Verification items for the finished model (mm, model axes). Face numbers are marked on the shaded views. Round coordinates to 2 decimals unless told otherwise and drop trailing zeros. Order: outer loops, then holes, each group sorted by start corner. A loop starts at its lowest first (then second) coordinate and runs counter-clockwise, first axis right, second up. Notation, with made-up numbers: M -11.75,-16.75 L 29.25,-16.75 A27 cw 29.25,22.25 Z; hole C 2,-24 d9. An arc over 180 degrees is marked long. Write item = value, one per line. Start each with the question number.
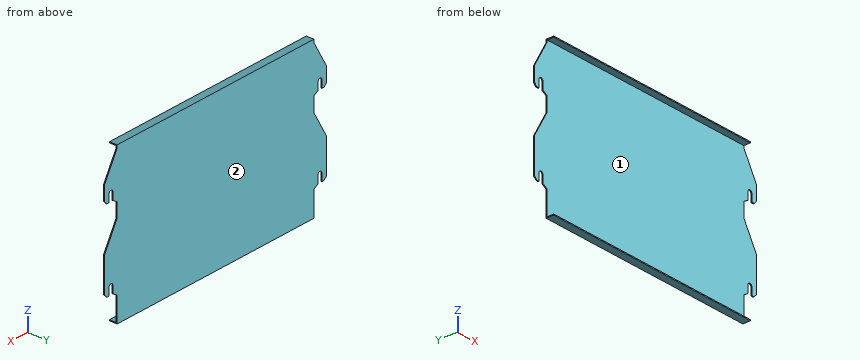
from build123d import *

# Parameters (mm, degrees)
EXTRUDE_THIN1_DEPTH = 132
CUT_EXTRUDE1_DEPTH  = 10


with BuildPart() as part:
    # Sketch1 → Extrude-Thin1 (new, symmetric)
    with BuildSketch(Plane(origin=(0, 0, 0), x_dir=(0, 0, -1), z_dir=(1, 0, 0))):
        Polygon((-80.5, -8), (-80.5, 0), (80.5, 0), (80.5, -8), (79.5, -8), (79.5, -1), (-79.5, -1), (-79.5, -8), align=None)
    extrude(amount=EXTRUDE_THIN1_DEPTH, both=True)

    # Sketch2 → Cut-Extrude1 (cut)
    with BuildSketch(Plane(origin=(0, 0, 0), x_dir=(1, 0, 0), z_dir=(0, 1, 0))):
        with BuildLine():
            Line((-117, 80.5), (-117, 54.5))
            Line((-117, 54.5), (-122, 51.5))
            Line((-122, 51.5), (-122, 43.5))
            ThreePointArc((-122, 43.5), (-124.25, 41.25), (-126.5, 43.5))
            Line((-126.5, 43.5), (-126.5, 51.5))
            Line((-126.5, 51.5), (-129, 51.5))
            Line((-129, 51.5), (-132, 48.5))
            Line((-132, 48.5), (-132, 12.5))
            Line((-132, 12.5), (-117, -14.5))
            Line((-117, -14.5), (-117, -29.5))
            Line((-117, -29.5), (-122, -32.5))
            Line((-122, -32.5), (-122, -40.5))
            ThreePointArc((-122, -40.5), (-124.25, -42.75), (-126.5, -40.5))
            Line((-126.5, -40.5), (-126.5, -32.5))
            Line((-126.5, -32.5), (-129.5, -32.5))
            Line((-129.5, -32.5), (-132, -35.5))
            Line((-132, -35.5), (-132, -50.5))
            Line((-132, -50.5), (-117, -77.5))
            Line((-117, -77.5), (-117, -80.5))
            Line((-117, -80.5), (-140, -80.5))
            Line((-140, -80.5), (-140, 80.5))
            Line((-140, 80.5), (-117, 80.5))
        make_face()
    cut_extrude1 = extrude(amount=-CUT_EXTRUDE1_DEPTH, mode=Mode.SUBTRACT)

    # Mirror1: Cut-Extrude1 across plane
    add(cut_extrude1.mirror(Plane(origin=(0, 0, 0), x_dir=(0, 0, 1), z_dir=(1, 0, 0))), mode=Mode.SUBTRACT)


solid = part.part
1) Scan lines: probe 1 along Z at (x, y) = (-25, -2.25); probe 2 along Y at (x, z) = (110.5, -18.5). Record each from-to range of solid material in increasing order.
2) Cross-section at B-B, the plane x = -28.5. Enter the section's corners in (y, z), then the cut area to 3 significant figures.
3) Cross-section at D-D, the plane z = -38. Enter the section's corners in (x, y), then the cut area to 3 significant figures.
4) Gauge pin test, flat ends, axial feed: P1, Ø5, axis at x = -89, z = -31.5, coming from the +Y side; P2, Ø3.5, axis at y = -5, z = 79.5, coming from the -X side; P3, Ø1.1, axis at y = -0.5, z = 23, coming from the +X side; P4, Ø0.5, axis at x = -128.5, y = -0.5, coming from the -Z side. Record the tip position at first contact, or that the pin passes through.
5) Cross-section at A-A, the plane y = -5.25. Enter the section's corners in (x, z), then the cut area to 3 significant figures.
6) Cross-section at C-C, the plane z = -67. Enter the section's corners in (x, y).
7) Release check for a two-part mould opening along Z. For the marked faces 1 and 2 record: pulls with the +Z half, pulls with the -Z half, needs draft (parallel to the pull), parting line crosses it, or undercut.
Geometry results:
q1.probe_1 = -80.5 to -79.5, 79.5 to 80.5
q1.probe_2 = -1 to 0
q2.outline = M -8,-80.5 L 0,-80.5 L 0,80.5 L -8,80.5 L -8,79.5 L -1,79.5 L -1,-79.5 L -8,-79.5 Z
q2.area = 175 mm^2
q3.outline = M -132,-1 L 132,-1 L 132,0 L -132,0 Z
q3.area = 264 mm^2
q4.P1 = 0
q4.P2 = -117
q4.P3 = 117
q4.P4 = -51.5
q5.outline = M -117,-80.5 L 117,-80.5 L 117,-79.5 L -117,-79.5 Z; M -117,79.5 L 117,79.5 L 117,80.5 L -117,80.5 Z
q5.area = 468 mm^2
q6.outline = M -117,-1 L 117,-1 L 117,0 L -117,0 Z
q7.face_1 = undercut
q7.face_2 = needs draft
